from build123d import *

# Parameters (mm, degrees)
SKETCH2_W          = 1.835
SKETCH2_H          = 1.03
SKETCH2_W_2        = 1.03
SKETCH2_H_2        = 1.835
CUT_EXTRUDE1_DEPTH = 2.74
CHAMFER1_SIZE      = 0.4
DRAFT1_ANGLE       = 26.5


with BuildPart() as part:
    # Sketch1 → Revolve1 (revolve)
    with BuildSketch(Plane.XY):
        with BuildLine():
            Line((-43.7, 0), (-43.7, 2.5))
            Line((-43.7, 2.5), (-3.7, 2.5))
            Line((-3.7, 2.5), (-3.7, 4.75))
            Line((-3.7, 4.75), (-1.562803405, 4.75))
            ThreePointArc((-1.562803405, 4.75), (-0.400737774, 2.500242712), (0, 0))
            Line((0, 0), (-43.7, 0))
        make_face()
    revolve(axis=Axis((0, 0, 0), (-1, 0, 0)))

    # Sketch2 → Cut-Extrude1 (cut)
    with BuildSketch(Plane(origin=(0, 0, 0), x_dir=(0, 0, -1), z_dir=(1, 0, 0))):
        with Locations((-1.4325, 0)):
            Rectangle(SKETCH2_W, SKETCH2_H)
        with Locations((0, 1.4325)):
            Rectangle(SKETCH2_W_2, SKETCH2_H_2)
        Rectangle(SKETCH2_W_2, SKETCH2_H)
        with Locations((0, -1.4325)):
            Rectangle(SKETCH2_W_2, SKETCH2_H_2)
        with Locations((1.4325, 0)):
            Rectangle(SKETCH2_W, SKETCH2_H)
    extrude(amount=-CUT_EXTRUDE1_DEPTH, mode=Mode.SUBTRACT)

    # Chamfer1
    chamfer1_edges = [part.edges().sort_by_distance(p)[0] for p in [
        (-43.7, -2.5, 0),
    ]]
    chamfer(chamfer1_edges, length=CHAMFER1_SIZE)

    # Draft1
    draft1_faces = [part.faces().sort_by_distance(p)[0] for p in [
        (-1.549357489, 0, -2.35),
        (-1.549357489, -2.35, 0),
        (-1.549357489, 2.35, 0),
        (-1.549357489, 0, 2.35),
    ]]
    draft(draft1_faces, Plane(origin=(0, 0, 0), x_dir=(0, 0, 1), z_dir=(1, 0, 0)), DRAFT1_ANGLE)


solid = part.part
Here's how the part is built. I have some questions about the finished solid (model axes, mm). A direction names the side the tool comes from. Round coordinates to 2 decimals unless told otherwise and drop trailing zeros. Loops run counter-clockwise (first coordinate to the right, second up) from the corner with the lowest first, then second, coordinate; pieces in that order, holes last.
1. Which directions (+Z, -Z, +X, -X, +Y, -Y) give clear straight access to the entire face, cutting with the end or side of a thin tool? Please do faces 1 (the face through (-23.22, -0.54, 2.44)), 2 (the face through (-1, 1, 0.515)).
Answer list:
face 1: -X
face 2: +X
2. For P1, Ø1.5, axis at x = -7, z = -0.5, coming from the -Y side; P2, Ø1.3, axis at x = -1, y = -1, coming from the +Z side; P3, Ø0.5, axis at x = -1.5, y = -1.5, coming from the -Z side, each with a flat end and sliding along its axis, tell me the tip position at first contact or that it passes through.
Answer list:
P1: stops at y = -2.5
P2: stops at z = 4.7
P3: stops at z = -4.58
3. We'd pull the mould along Y, two halves only. Please class faces 3 (the face through (-1, -0.515, 1)), 4 (the face through (-43.7, 0, 0)), 5 (the face through (-2.616, 2.192, 4.214)): +Y half, -Y half, draft (parallel to the pull), parting line (faces both ways), or undercut.
Answer list:
face 3: undercut
face 4: draft
face 5: parting line
4. If I drill on line 1 along Z through (x, y) = (-8, 0); line 2 along Y through (x, z) = (-15, -1.75); line 3 along X through (y, z) = (3.75, 0.25), over which ranges is the centre line in solid material (lowest first)?
Answer list:
line 1: z = -2.5 to 2.5
line 2: y = -1.79 to 1.79
line 3: x = -3.7 to -0.94
5. If we section it at D-D on z = 4: Write out the boundary of the cut face in (x, y), plus the area to 3 significant figures.
Answer list:
outline: (-3.7, -2.56) - (-1.56, -2.56) arc R6.93 ccw to (-1.56, 2.56) - (-3.7, 2.56) - close
area: 12.6 mm2
6. If we section it at A-A on z = 0: Write out the boundary of the cut face in (x, y).
Answer list:
outline: (-43.7, -2.1) - (-43.3, -2.5) - (-3.7, -2.5) - (-3.7, -4.75) - (-1.56, -4.75) arc R8 ccw to (-0.31, -2.2) - (-2.74, -0.98) - (-2.74, 0.98) - (-0.31, 2.2) arc R8 ccw to (-1.56, 4.75) - (-3.7, 4.75) - (-3.7, 2.5) - (-43.3, 2.5) - (-43.7, 2.1) - close
7. If we section it at C-C on x = -16: Write out the boundary of the cut face in (y, z).
Answer list:
outline: circle Ø5 at (0, 0)
